Design review of the part built by this model. Coordinates are the model's own, in mm. A direction names the side the tool comes from. Round coordinates to 2 decimals unless told otherwise and drop trailing zeros. Write each loop counter-clockwise with the first axis right and the second up, starting at its lowest first coordinate (ties: lowest second). Pieces come first, ordered by that corner, then holes. Notation, with made-up numbers: (26.5, 77.25) -> (61.5, 77.25) arc R31 cw to (61.5, 109.25) -> close; hole circle Ø7 at (9.5, -11.75). An arc over 180 degrees is marked (long way). One line per question, with ' | ' between items. Start each with the question number.
1) Insertion check: pin 1 Ø5 at (y, z) = (-3, 35) entering from -X; pin 2 Ø2.5 at (y, z) = (-6.5, 77) entering from -X; pin 3 Ø12 at (x, z) = (-17, 63) entering from +Y. Each pin has a flat end and moves straight along its axis. Give the tip position at first contact, or say it passes through.
2) Mouldability with a two-part tool opening along X and no side actions: class faces 4 (the flat face through (34, -9, 65)), 5 (the flat face through (24, -6, 80)) as +X half, -X half, draft (parallel to the pull), parting line (faces both ways), or undercut.
3) Consider section C-C (y = -2). Give the boundary of the cut face in (x, z).
4) For faces 1 (the cylindrical face through (15.78, -19.77, 14.74)), 2 (the flat face through (69, -19, 75)), 3 (the flat face through (-39, -6, 80)), list the 3-axis set-ups (+Z, -Z, +X, -X, +Y, -Y) from which the entire face can be reached by the end or side of a thin tool; tool diameter is ignored.
5) For probe 1 along X at (y, z) = (-11.5, 54); probe 2 along X at (y, z) = (12, 60.5); probe 3 along Y at (x, z) = (-39.5, 6), list the stretches that pass through material, from the lowest coordinate up.
6) Consider section D-D (x = 68.5). Give the boundary of the cut face in (y, z).
7) Consider section A-A (z = 17). Give the boundary of the cut face in (x, y) (3 decimals).
8) Consider section B-B (x = 0). Give the boundary of the cut face in (y, z) (3 decimals).
```python
from build123d import *

# Parameters (mm, degrees)
F1_DEPTH     = 100
F0_R         = 14
F2_DEPTH     = 50
F3_DEPTH     = 75
F4_DEPTH     = 85
F0_W         = 5
F0_H         = 5
F5_DEPTH     = 80
F6_START     = 25
F0_W_2       = 28
F0_H_2       = 3.9854568298
F6_DEPTH     = 25
F7_START     = 75
F0_W_3       = 9
F0_H_3       = 7
F0_H_4       = 6
F7_DEPTH     = 25
F8_DEPTH     = 60
F9_T1_DEPTH  = 28
F9_T3_DEPTH  = 37.2399709343
F9_T9_DEPTH  = 40.2399709343
F9_T13_DEPTH = 37.2399709343
F9_T20_DEPTH = 37.2399709343
F9_T24_DEPTH = 40.2399709343
F10_START    = 65
F0_W_4       = 3
F10_DEPTH    = 10
F11_DEPTH    = 60


# Not quite as in the source:
# - a fillet or chamfer that OpenCascade refuses, or shapes differently, is made with other operations: its cross-section is extruded or revolved along the edge and cut away or added
# - a feature names something its author has since deleted; it is built from what else it names


with BuildPart() as f1:
    # F0 (on Top) → F1 (new body)
    with BuildSketch(Plane.XY):
        with BuildLine():
            ThreePointArc((-49.982315052, -12), (-47.3993365724, -6.2454186413), (-46.5151813626, 0))
            ThreePointArc((-46.5151813626, 0), (-47.3993365724, 6.2454186413), (-49.982315052, 12))
            ThreePointArc((-49.982315052, 12), (-87.5239224573, 12.7936118078), (-73.5151813626, -22.045407685))
            Line((-73.5151813626, -22.045407685), (-73.5151813626, -15.045407685))
            Line((-73.5151813626, -15.045407685), (-64.5151813626, -15.045407685))
            Line((-64.5151813626, -15.045407685), (-64.5151813626, -22.045407685))
            ThreePointArc((-64.5151813626, -22.045407685), (-56.2215695548, -18.5087410947), (-49.982315052, -12))
        make_face()
    extrude(amount=F1_DEPTH)



with BuildPart() as f1b:
    # F0 (on Top) → F1, piece 2 (new body)
    with BuildSketch(Plane.XY):
        with BuildLine():
            ThreePointArc((49.982315052, 12), (47.3993365677, 6.2454186249), (46.5151813626, -3.41e-08))
            ThreePointArc((46.5151813626, -3.41e-08), (47.3993365771, -6.2454186577), (49.982315052, -12))
            ThreePointArc((49.982315052, -12), (56.2215695548, -18.5087410947), (64.5151813626, -22.045407685))
            Line((64.5151813626, -22.045407685), (64.5151813626, -16.045407685))
            Line((64.5151813626, -16.045407685), (73.5151813626, -16.045407685))
            Line((73.5151813626, -16.045407685), (73.5151813626, -22.045407685))
            ThreePointArc((73.5151813626, -22.045407685), (86.4436064206, -14.2302494708), (91.5151813626, 0))
            ThreePointArc((91.5151813626, 0), (75.2606000039, 21.6158447902), (49.982315052, 12))
        make_face()
    extrude(amount=F1_DEPTH)


with BuildPart() as f1_1:
    add(f1.part)

    add(f1b.part)  # F2 merges F1b
    # F0 (on Top) → F2 (join)
    with BuildSketch(Plane.XY):
        Polygon((46.5151813626, 12), (46.5151813626, 20.8604575003), (-46.5151813626, 20.8604575003), (-46.5151813626, 12), (-46.5151813626, 0), (-46.5151813626, -12), (-46.5151813626, -20.8604575003), (-14.0001813626, -20.8604575003), (-14.0001813626, -16.8750006706), (13.9998186374, -16.8750006706), (13.9998186374, -20.8604575003), (46.5151813626, -20.8604575003), (46.5151813626, -12), (46.5151813626, -3.41e-08), align=None)
        Polygon((-26.5151813626, 9), (-21.5151813626, 9), (-21.5151813626, 4), (-21.5151813626, -4), (-21.5151813626, -9), (-26.5151813626, -9), (-30.1052076072, -9), (-33.1052076072, -9), (-36.5151813626, -9), (-41.5151813626, -9), (-41.5151813626, -4), (-41.5151813626, 4), (-41.5151813626, 9), (-36.5151813626, 9), align=None, mode=Mode.SUBTRACT)
        Circle(F0_R, mode=Mode.SUBTRACT)
        Polygon((36.9421700871, 9), (41.9421700871, 9), (41.9421700871, 4), (41.9421700871, -4), (41.9421700871, -9), (36.9421700871, -9), (33.5321700871, -9), (30.5321700871, -9), (26.9421700871, -9), (21.9421700871, -9), (21.9421700871, -4), (21.9421700871, 4), (21.9421700871, 9), (26.9421700871, 9), align=None, mode=Mode.SUBTRACT)
        with BuildLine():
            Line((-46.5151813626, -12), (-46.5151813626, 0))
            ThreePointArc((-46.5151813626, 0), (-47.3993365724, -6.2454186413), (-49.982315052, -12))
            Line((-49.982315052, -12), (-46.5151813626, -12))
        make_face()
        with BuildLine():
            Line((-46.5151813626, 0), (-46.5151813626, 12))
            Line((-46.5151813626, 12), (-49.982315052, 12))
            ThreePointArc((-49.982315052, 12), (-47.3993365724, 6.2454186413), (-46.5151813626, 0))
        make_face()
        with BuildLine():
            ThreePointArc((49.982315052, -12), (47.3993365771, -6.2454186577), (46.5151813626, -3.41e-08))
            Line((46.5151813626, -3.41e-08), (46.5151813626, -12))
            Line((46.5151813626, -12), (49.982315052, -12))
        make_face()
        with BuildLine():
            Line((49.982315052, 12), (46.5151813626, 12))
            Line((46.5151813626, 12), (46.5151813626, -3.41e-08))
            ThreePointArc((46.5151813626, -3.41e-08), (47.3993365677, 6.2454186249), (49.982315052, 12))
        make_face()
    extrude(amount=F2_DEPTH)

    # F0 (on Top) → F3 (join)
    with BuildSketch(Plane.XY):
        Polygon((36.9421700871, 4), (36.9421700871, 9), (26.9421700871, 9), (26.9421700871, 4), (21.9421700871, 4), (21.9421700871, -4), (26.9421700871, -4), (26.9421700871, -9), (30.5321700871, -9), (30.5321700871, -4), (33.5321700871, -4), (33.5321700871, -9), (36.9421700871, -9), (36.9421700871, -4), (41.9421700871, -4), (41.9421700871, 4), align=None)
        Polygon((-26.5151813626, 4), (-26.5151813626, 9), (-36.5151813626, 9), (-36.5151813626, 4), (-41.5151813626, 4), (-41.5151813626, -4), (-36.5151813626, -4), (-36.5151813626, -9), (-33.1052076072, -9), (-33.1052076072, -4), (-30.1052076072, -4), (-30.1052076072, -9), (-26.5151813626, -9), (-26.5151813626, -4), (-21.5151813626, -4), (-21.5151813626, 4), align=None)
    extrude(amount=F3_DEPTH)

    # F0 (on Top) → F4 (join)
    with BuildSketch(Plane.XY):
        Circle(F0_R)
    extrude(amount=F4_DEPTH)

    # F0 (on Top) → F5 (join)
    with BuildSketch(Plane.XY):
        with Locations((-39.0151813626, 6.5)):
            Rectangle(F0_W, F0_H)
        with Locations((-39.0151813626, -6.5)):
            Rectangle(F0_W, F0_H)
        with Locations((-24.0151813626, -6.5)):
            Rectangle(F0_W, F0_H)
        with Locations((-24.0151813626, 6.5)):
            Rectangle(F0_W, F0_H)
        with Locations((24.4421700871, -6.5)):
            Rectangle(F0_W, F0_H)
        with Locations((39.4421700871, -6.5)):
            Rectangle(F0_W, F0_H)
        with Locations((39.4421700871, 6.5)):
            Rectangle(F0_W, F0_H)
        with Locations((24.4421700871, 6.5)):
            Rectangle(F0_W, F0_H)
    extrude(amount=F5_DEPTH)

    # F0 (on Top) → F6 (join)
    with BuildSketch(Plane.XY.offset(F6_START)):
        with Locations((-0.0001813626, -18.8677290854)):
            Rectangle(F0_W_2, F0_H_2)
    extrude(amount=F6_DEPTH)

    # F0 (on Top) → F7 (join)
    with BuildSketch(Plane.XY.offset(F7_START)):
        with Locations((-69.0151813626, -18.545407685)):
            Rectangle(F0_W_3, F0_H_3)
        with Locations((69.0151813626, -19.045407685)):
            Rectangle(F0_W_3, F0_H_4)
    extrude(amount=F7_DEPTH)

    # F0 (on Top) → F8 (join)
    with BuildSketch(Plane.XY):
        with Locations((-69.0151813626, -18.545407685)):
            Rectangle(F0_W_3, F0_H_3)
        with Locations((69.0151813626, -19.045407685)):
            Rectangle(F0_W_3, F0_H_4)
    extrude(amount=F8_DEPTH)

    # F9: fillet of radius 5 on 3 edges, made by hand

    # F9_s2 → F9_t1 (cut)
    with BuildSketch(Plane.YZ.offset(-14.0001813626)):
        with BuildLine():
            ThreePointArc((-20.8604575003, 29.8959883737), (-19.7381317937, 26.7394646412), (-16.8750006706, 25))
            Line((-16.8750006706, 25), (-20.8604575003, 25))
            Line((-20.8604575003, 25), (-20.8604575003, 29.8959883737))
        make_face()
    extrude(amount=F9_T1_DEPTH, mode=Mode.SUBTRACT)

    # F9_s4 → F9_t3 (cut)
    with BuildSketch(Plane.XY.offset(-12.2399709343)):
        with BuildLine():
            ThreePointArc((-18.8961697364, -20.8604575003), (-15.7396460038, -19.7381317937), (-14.0001813626, -16.8750006706))
            Line((-14.0001813626, -16.8750006706), (-14.0001813626, -20.8604575003))
            Line((-14.0001813626, -20.8604575003), (-18.8961697364, -20.8604575003))
        make_face()
        with BuildLine():
            ThreePointArc((18.8958070111, -20.8604575003), (15.7392832785, -19.7381317937), (13.9998186374, -16.8750006706))
            Line((13.9998186374, -16.8750006706), (13.9998186374, -20.8604575003))
            Line((13.9998186374, -20.8604575003), (18.8958070111, -20.8604575003))
        make_face()
    extrude(amount=F9_T3_DEPTH, mode=Mode.SUBTRACT)


with BuildPart() as f9_tool7:
    # F9_s8 → F9_t9 (new body)
    with BuildSketch(Plane.YZ.offset(-26.240152297)):
        with BuildLine():
            ThreePointArc((-20.8604575003, 29.8959883737), (-19.7381317937, 26.7394646412), (-16.8750006706, 25))
            Line((-16.8750006706, 25), (-20.8604575003, 25))
            Line((-20.8604575003, 25), (-20.8604575003, 29.8959883737))
        make_face()
    extrude(amount=F9_T9_DEPTH)

    split(bisect_by=Plane.YZ.offset(-14.0001813626), keep=Keep.BOTTOM)


with BuildPart() as f9_tool11:
    # F9_s12 → F9_t13 (new body)
    with BuildSketch(Plane.XY):
        with BuildLine():
            ThreePointArc((-18.8961697364, -20.8604575003), (-15.7396460038, -19.7381317937), (-14.0001813626, -16.8750006706))
            Line((-14.0001813626, -16.8750006706), (-14.0001813626, -20.8604575003))
            Line((-14.0001813626, -20.8604575003), (-18.8961697364, -20.8604575003))
        make_face()
    extrude(amount=F9_T13_DEPTH)

    split(bisect_by=Plane.XY.offset(25), keep=Keep.TOP)


with BuildPart() as f9_tool7_1:
    add(f9_tool7.part)

    # F9_t15: intersect F9_tool11
    add(f9_tool11.part, mode=Mode.INTERSECT)


with BuildPart() as f1_2:
    add(f1_1.part)

    # F9_t5: cut F9_tool7
    add(f9_tool7_1.part, mode=Mode.SUBTRACT)


with BuildPart() as f9_tool18:
    # F9_s19 → F9_t20 (new body)
    with BuildSketch(Plane.XY):
        with BuildLine():
            ThreePointArc((18.8958070111, -20.8604575003), (15.7392832785, -19.7381317937), (13.9998186374, -16.8750006706))
            Line((13.9998186374, -16.8750006706), (13.9998186374, -20.8604575003))
            Line((13.9998186374, -20.8604575003), (18.8958070111, -20.8604575003))
        make_face()
    extrude(amount=F9_T20_DEPTH)

    split(bisect_by=Plane.XY.offset(25), keep=Keep.TOP)


with BuildPart() as f9_tool22:
    # F9_s23 → F9_t24 (new body)
    with BuildSketch(Plane.YZ.offset(-14.0001813626)):
        with BuildLine():
            ThreePointArc((-20.8604575003, 29.8959883737), (-19.7381317937, 26.7394646412), (-16.8750006706, 25))
            Line((-16.8750006706, 25), (-20.8604575003, 25))
            Line((-20.8604575003, 25), (-20.8604575003, 29.8959883737))
        make_face()
    extrude(amount=F9_T24_DEPTH)

    split(bisect_by=Plane.YZ.offset(13.9998186374), keep=Keep.TOP)


with BuildPart() as f9_tool18_1:
    add(f9_tool18.part)

    # F9_t26: intersect F9_tool22
    add(f9_tool22.part, mode=Mode.INTERSECT)


with BuildPart() as f1_3:
    add(f1_2.part)

    # F9_t16: cut F9_tool18
    add(f9_tool18_1.part, mode=Mode.SUBTRACT)

    # F0 (on Top) → F10 (join)
    with BuildSketch(Plane.XY.offset(F10_START)):
        with Locations((-31.6052076072, -6.5)):
            Rectangle(F0_W_4, F0_H)
        with Locations((32.0321700871, -6.5)):
            Rectangle(F0_W_4, F0_H)
    extrude(amount=F10_DEPTH)

    # F0 (on Top) → F11 (join)
    with BuildSketch(Plane.XY):
        with Locations((-31.6052076072, -6.5)):
            Rectangle(F0_W_4, F0_H)
        with Locations((32.0321700871, -6.5)):
            Rectangle(F0_W_4, F0_H)
    extrude(amount=F11_DEPTH)


solid = f1_3.part
```
From the geometry:
1) pin 1: stops at x = -91.51 | pin 2: stops at x = -90.89 | pin 3: stops at y = 9
2) face 4: undercut | face 5: undercut
3) outline: (-91.43, 0) -> (91.43, 0) -> (91.43, 100) -> (46.6, 100) -> (46.6, 50) -> (41.94, 50) -> (41.94, 75) -> (21.94, 75) -> (21.94, 50) -> (13.86, 50) -> (13.86, 85) -> (-13.86, 85) -> (-13.86, 50) -> (-21.52, 50) -> (-21.52, 75) -> (-41.52, 75) -> (-41.52, 50) -> (-46.6, 50) -> (-46.6, 100) -> (-91.43, 100) -> close
4) face 1: -Z, -Y | face 2: -Y | face 3: +Z, +Y, -Y
5) probe 1: x = -88.35 to -49.68, -7.98 to 7.98, 49.68 to 88.35 | probe 2: x = -88.05 to -49.98, -7.21 to 7.21, 49.98 to 88.05 | probe 3: y = -20.86 to 20.86
6) outline: (-22.05, 0) -> (22.49, 0) -> (22.49, 100) -> (-22.05, 100) -> (-22.05, 75) -> (-16.05, 75) -> (-16.05, 60) -> (-22.05, 60) -> close
7) outline: (-73.515, -22.045) -> (-64.515, -22.045) arc R22.5 ccw to (-49.982, -12) -> (-46.515, -12) -> (-46.515, -20.86) -> (-18.896, -20.86) arc R5 ccw to (-14, -16.875) -> (14, -16.875) arc R5 ccw to (18.896, -20.86) -> (46.515, -20.86) -> (46.515, -12) -> (49.982, -12) arc R22.5 ccw to (64.515, -22.045) -> (73.515, -22.045) arc R22.5 ccw (long way) to (49.982, 12) -> (46.515, 12) -> (46.515, 20.86) -> (-46.515, 20.86) -> (-46.515, 12) -> (-49.982, 12) arc R22.5 ccw (long way) to start
8) outline: (-20.86, 29.896) arc R5 ccw to (-16.875, 25) -> (-16.875, 0) -> (20.86, 0) -> (20.86, 50) -> (14, 50) -> (14, 85) -> (-14, 85) -> (-14, 50) -> (-20.86, 50) -> close
